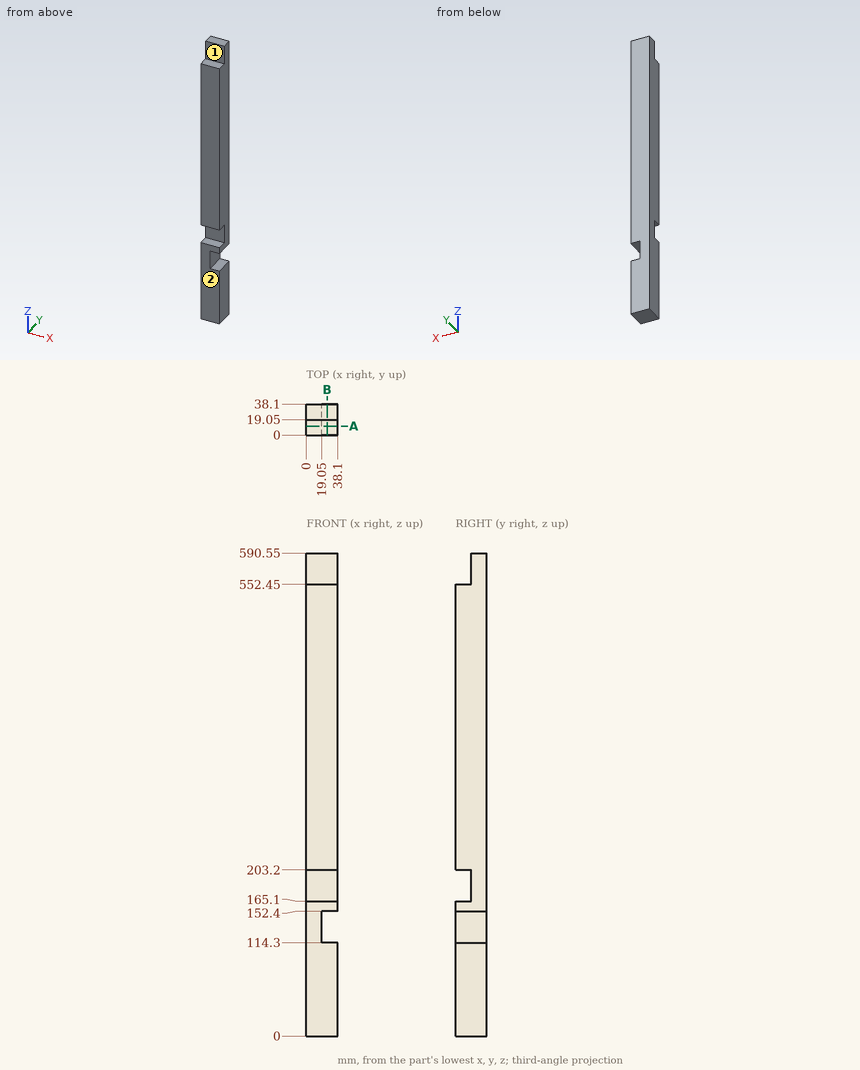
For this review, use the dimensioned drawing (mm, ordinates from the lowest corner) and the shaded views. A direction names the side the tool comes from. Round coordinates to 2 decimals unless told otherwise and drop trailing zeros. Order: outer loops, then holes, each group sorted by start corner. A loop starts at its lowest first (then second) coordinate and runs counter-clockwise, first axis right, second up. Notation, with made-up numbers: (-17, 41) -> (23, 41) arc R20 ccw to (23, 55) -> close; hole circle Ø6 at (89, -24). An arc over 180 degrees is marked (long way). One line per item, written item: value. Start each with the question number.
Q1. Machinability: for the marked faces 1 and 2, which of the approach directions +Z, -Z, +X, -X, +Y, -Y give a long, thin tool a straight path to every point of the face, cutting with its end or side? Answer none if there is none.
Q2. Clearance check with flat-ended pins moving along their axes: pin 1 Ø11.5 at (x, z) = (24.5, 184) entering from -Y; pin 2 Ø9.5 at (x, y) = (17.5, 9) entering from +Z. State where each tip first meets the part, or that it passes through.
Q3. Take a section at B-B (x = 25.5). Write out the cut boundary in (y, z), and give its area (3 significant figures).
Q4. Take a section at A-A (y = 11). Write out the cut boundary in (x, z).
Q5. Wall thickness on line 1 (Z direction, x = 20, y = 6.5); line 2 (Z direction, x = 21.5, y = 22); line 3 (Z direction, x = 3.5, y = 6.5): over which ranges is each line inside the solid? List them lowest first.
Reported:
1. face 1: +Z, +X, -X, -Y
1. face 2: +Z, -Z, +X, -X, -Y
2. pin 1: stops at y = 19.05
2. pin 2: stops at z = 552.45
3. outline: (0, 0) -> (38.1, 0) -> (38.1, 114.3) -> (0, 114.3) -> close; (0, 152.4) -> (38.1, 152.4) -> (38.1, 590.55) -> (19.05, 590.55) -> (19.05, 552.45) -> (0, 552.45) -> (0, 203.2) -> (19.05, 203.2) -> (19.05, 165.1) -> (0, 165.1) -> close
3. area: 19,600 mm2
4. outline: (0, 0) -> (38.1, 0) -> (38.1, 114.3) -> (19.05, 114.3) -> (19.05, 152.4) -> (38.1, 152.4) -> (38.1, 165.1) -> (0, 165.1) -> close; (0, 203.2) -> (38.1, 203.2) -> (38.1, 552.45) -> (0, 552.45) -> close
5. line 1: z = 0 to 114.3, 152.4 to 165.1, 203.2 to 552.45
5. line 2: z = 0 to 114.3, 152.4 to 590.55
5. line 3: z = 0 to 165.1, 203.2 to 552.45
